```python
from build123d import *

# Parameters (mm, degrees)
F0_W      = 41
F0_H      = 17
F0_W_2    = 20
F0_H_2    = 20
F1_DEPTH  = 20
F2_W      = 40.5264794827
F2_H      = 14.0749709308
F3_DEPTH  = 5
F4_W      = 25
F4_H      = 17.5813399255
F5_DEPTH  = 7
F6_W      = 20
F6_H      = 20
F7_DEPTH  = 5
F8_R      = 2
F9_DEPTH  = 10
F10_R     = 5
F11_DEPTH = 3
F12_W     = 35
F12_H     = 12.0767594278
F13_DEPTH = 17
F14_R     = 2
F15_DEPTH = 10


with BuildPart() as f1:
    # F0 (on Top) → F1 (new body)
    with BuildSketch(Plane.XY):
        with BuildLine():
            Line((-25, 21.15), (-25, -27.5))
            Line((-25, -27.5), (25, -27.5))
            Line((25, -27.5), (25, 21.15))
            ThreePointArc((25, 21.15), (23.1401280605, 25.6401280605), (18.65, 27.5))
            Line((18.65, 27.5), (-18.65, 27.5))
            ThreePointArc((-18.65, 27.5), (-23.1401280605, 25.6401280605), (-25, 21.15))
        make_face()
        with Locations((0, -16.5383797139)):
            Rectangle(F0_W, F0_H, mode=Mode.SUBTRACT)
        with Locations((0, 12.9625145346)):
            Rectangle(F0_W_2, F0_H_2, mode=Mode.SUBTRACT)
    extrude(amount=F1_DEPTH)

    # F2 (on face) → F3 (cut)
    with BuildSketch(Plane.XZ.offset(27.5)):
        with Locations((0, 12.9625145346)):
            Rectangle(F2_W, F2_H)
    extrude(amount=-F3_DEPTH, mode=Mode.SUBTRACT)

    # F4 (on face) → F5 (join)
    with BuildSketch(Plane(origin=(0, 0, 0), x_dir=(1, 0, 0), z_dir=(0, 0, -1))):
        with Locations((-37.5, 0)):
            Rectangle(F4_W, F4_H)
        with Locations((37.5, 0)):
            Rectangle(F4_W, F4_H)
    extrude(amount=-F5_DEPTH)

    # F6 (on face) → F7 (join)
    with BuildSketch(Plane.XY.offset(20)):
        with Locations((0, 12.9625145346)):
            Rectangle(F6_W, F6_H)
    extrude(amount=-F7_DEPTH)

    # F8 (on face) → F9 (cut)
    with BuildSketch(Plane.XY.offset(20)):
        with Locations((0, 14.1955753788)):
            Circle(F8_R)
    extrude(amount=-F9_DEPTH, mode=Mode.SUBTRACT)

    # F10 (on face) → F11 (cut)
    with BuildSketch(Plane.XY.offset(20)):
        with Locations((0, 14.1955753788)):
            Circle(F10_R)
    extrude(amount=-F11_DEPTH, mode=Mode.SUBTRACT)

    # F12 (on face) → F13 (cut)
    with BuildSketch(Plane.XY.offset(20)):
        Rectangle(F12_W, F12_H)
    extrude(amount=-F13_DEPTH, mode=Mode.SUBTRACT)

    # F14 (on face) → F15 (cut)
    with BuildSketch(Plane.XY.offset(7)):
        with Locations((-44, 0)):
            Circle(F14_R)
        with Locations((44, 0)):
            Circle(F14_R)
    extrude(amount=-F15_DEPTH, mode=Mode.SUBTRACT)


solid = f1.part
```
For this review, take the finished solid that the model builds, in its own axes (mm). A direction names the side the tool comes from. Coordinates: 2 decimals unless noted, no trailing zeros. Order: outer loops, then holes, each group sorted by start corner. A loop starts at its lowest first (then second) coordinate and runs counter-clockwise, first axis right, second up. Notation, with made-up numbers: (36, 73) -> (65, 73) arc R34 cw to (65, 109) -> close; hole circle Ø11 at (49, 42). An arc over 180 degrees is marked (long way). Use CSV: the item, a comma, the result in double quotes. Start each with the question number.
Item 1: We need section B-B, the plane z = 9. Give the boundary of the cut face in (x, y), then the cut area to 3 significant figures.
Item 2: Draft analysis for pull direction X (two halves, no side actions). For faces 4 (the face through (17.5, 0, 12)), 5 (the face through (37, 0, 7)), state which applies: pulls with the +X half, pulls with the -X half, needs draft (parallel to the pull), parting line crosses it, or undercut.
Item 3: Insertion check: pin 1 (3 mm diameter, centred on y = -18.5, z = 4.5, fed in from -X); pin 2 (2 mm diameter, centred on x = 35, z = 4.5, fed in from -Y); pin 3 (16 mm diameter, centred on x = 0, y = 14.2, fed in from -Z). Each pin has a flat end and moves straight along its axis. Give the tip position at first contact, or say it passes through.
Item 4: For faces 1 (the face through (0, -26, 5.925)), 2 (the face through (-0.2, 6.038, 15.4)), 3 (the face through (0, 22.963, 7)), list the 3-axis set-ups (+Z, -Z, +X, -X, +Y, -Y) from which the entire face can be reached by the end or side of a thin tool; tool diameter is ignored.
Item 5: We need section D-D, the plane x = -44. Give the boundary of the cut face in (y, z).
Item 6: We need section C-C, the plane y = -18. Give the boundary of the cut face in (x, z), then the cut area to 3 significant figures.
Item 7: We need section A-A, the plane y = 0. Give the boundary of the cut face in (x, z), then the cut area to 3 significant figures.
Item 8: Wall thickness on probe 1 along Y at (x, z) = (0, 15.5); probe 2 along Y at (x, z) = (0, 17.6); probe 3 along X at (y, z) = (-16, 10.5): over which ranges is each line inside the solid? List them lowest first.
Derived:
1,outline,"(-25, -27.5) -> (-20.26, -27.5) -> (-20.26, -25.04) -> (-20.5, -25.04) -> (-20.5, -8.04) -> (20.5, -8.04) -> (20.5, -25.04) -> (20.26, -25.04) -> (20.26, -27.5) -> (25, -27.5) -> (25, 21.15) arc R6.35 ccw to (18.65, 27.5) -> (-18.65, 27.5) arc R6.35 ccw to (-25, 21.15) -> close; hole (-17.5, -6.04) -> (17.5, -6.04) -> (17.5, 6.04) -> (10, 6.04) -> (10, 22.96) -> (-10, 22.96) -> (-10, 6.04) -> (-17.5, 6.04) -> close"
1,area,"1,170 mm^2"
2,face 4,"undercut"
2,face 5,"needs draft"
3,pin 1,"stops at x = -25"
3,pin 2,"stops at y = -8.79"
3,pin 3,"stops at z = 15"
4,face 1,"+Z, -Y"
4,face 2,"+Z"
4,face 3,"-Z"
5,outline,"(-8.79, 0) -> (-2, 0) -> (-2, 7) -> (-8.79, 7) -> close; (2, 0) -> (8.79, 0) -> (8.79, 7) -> (2, 7) -> close"
6,outline,"(-25, 0) -> (-20.5, 0) -> (-20.5, 20) -> (-25, 20) -> close; (20.5, 0) -> (25, 0) -> (25, 20) -> (20.5, 20) -> close"
6,area,"180 mm^2"
7,outline,"(-50, 0) -> (-46, 0) -> (-46, 7) -> (-50, 7) -> close; (-42, 0) -> (42, 0) -> (42, 7) -> (25, 7) -> (25, 20) -> (17.5, 20) -> (17.5, 3) -> (-17.5, 3) -> (-17.5, 20) -> (-25, 20) -> (-25, 7) -> (-42, 7) -> close; (46, 0) -> (50, 0) -> (50, 7) -> (46, 7) -> close"
7,area,"699 mm^2"
8,probe 1,"y = -8.04 to -6.04, 6.04 to 12.2, 16.2 to 27.5"
8,probe 2,"y = -8.04 to -6.04, 6.04 to 9.2, 19.2 to 27.5"
8,probe 3,"x = -25 to -20.5, 20.5 to 25"
